Input: part model. Units: mm. Frame: model coordinates. Round coordinates to 2 decimals unless told otherwise and drop trailing zeros. Order: outer loops, then holes, each group sorted by start corner. A loop starts at its lowest first (then second) coordinate and runs counter-clockwise, first axis right, second up. Notation, with made-up numbers: (60.25, 75.25) -> (98.25, 75.25) arc R14 cw to (98.25, 79.25) -> close; hole circle Ø3 at (79, 7). An arc over 180 degrees is marked (long way). Use a Markdown table: item, result.
from build123d import *

# Parameters (mm, degrees)
F0_W     = 228.6
F0_H     = 177.8
F1_DEPTH = 3.175
F2_R     = 5.08


with BuildPart() as f1:
    # F0 (on Top) → F1 (new body)
    with BuildSketch(Plane.XY):
        with Locations((-0.871601, -3.897959)):
            Rectangle(F0_W, F0_H)
        Polygon((-35.42317, -63.4338), (-80.133474, -63.4338), (-56.54095, -14.745583), align=None, mode=Mode.SUBTRACT)
        Polygon((23.823941, -63.4338), (-13.718781, -63.4338), (4.465975, -14.745583), align=None, mode=Mode.SUBTRACT)
        Polygon((80.13803, -63.4338), (42.118688, -63.4338), (57.847038, -15.083696), align=None, mode=Mode.SUBTRACT)
        with BuildLine():
            Line((-90.692364, -63.4338), (-90.692364, 57.993443))
            Line((-90.692364, 57.993443), (-67.099841, 19.27751))
            ThreePointArc((-67.099841, 19.27751), (-62.324984, 2.265963), (-67.099841, -14.745583))
            Line((-67.099841, -14.745583), (-90.692364, -63.4338))
        make_face(mode=Mode.SUBTRACT)
        with BuildLine():
            ThreePointArc((-46.568668, -14.745583), (-50.040228, 2.291953), (-46.322669, 19.27751))
            Line((-46.322669, 19.27751), (-24.523671, 57.993443))
            Line((-24.523671, 57.993443), (-7.852732, 19.27751))
            ThreePointArc((-7.852732, 19.27751), (-4.872698, 2.265963), (-7.852732, -14.745583))
            Line((-7.852732, -14.745583), (-25.450888, -63.4338))
            Line((-25.450888, -63.4338), (-46.568668, -14.745583))
        make_face(mode=Mode.SUBTRACT)
        Polygon((-56.54095, 19.27751), (-80.133474, 57.993443), (-34.060732, 57.993443), align=None, mode=Mode.SUBTRACT)
        with BuildLine():
            Line((49.04796, -14.745583), (33.209621, -63.4338))
            Line((33.209621, -63.4338), (13.851655, -14.745583))
            ThreePointArc((13.851655, -14.745583), (10.593866, 2.265963), (13.851655, 19.27751))
            Line((13.851655, 19.27751), (33.31961, 57.993443))
            Line((33.31961, 57.993443), (49.04796, 19.27751))
            ThreePointArc((49.04796, 19.27751), (51.745333, 2.265963), (49.04796, -14.745583))
        make_face(mode=Mode.SUBTRACT)
        Polygon((4.465975, 19.27751), (-14.891991, 57.993443), (23.823941, 57.993443), align=None, mode=Mode.SUBTRACT)
        with BuildLine():
            Line((66.646114, 19.27751), (88.937106, 57.993443))
            Line((88.937106, 57.993443), (88.937106, -63.4338))
            Line((88.937106, -63.4338), (69.157515, -14.745583))
            ThreePointArc((69.157515, -14.745583), (65.224515, 2.06834), (66.646114, 19.27751))
        make_face(mode=Mode.SUBTRACT)
        Polygon((57.847038, 19.27751), (42.118688, 57.993443), (80.13803, 57.993443), align=None, mode=Mode.SUBTRACT)
    extrude(amount=F1_DEPTH)

    # F2
    f2_edges = [f1.edges().sort_by_distance(p)[0] for p in [
        (-90.692364, -63.4338, 1.5875),
        (-90.692364, 57.993443, 1.5875),
    ]]
    fillet(f2_edges, radius=F2_R)


solid = f1.part
1) Cut plane B-B on x = 2. Return loops of the section in (y, z) (3 decimals).
Answer key:
| item | result |
|---|---|
| outline | (-92.798, 0) -> (-63.434, 0) -> (-63.434, 3.175) -> (-92.798, 3.175) -> close; (-21.348, 0) -> (24.209, 0) -> (24.209, 3.175) -> (-21.348, 3.175) -> close; (57.993, 0) -> (85.002, 0) -> (85.002, 3.175) -> (57.993, 3.175) -> close |
2) Cut plane C-C on y = 13. Return loops of the section in (x, z) (3 decimals).
Answer key:
| item | result |
|---|---|
| outline | (-115.172, 0) -> (-90.692, 0) -> (-90.692, 3.175) -> (-115.172, 3.175) -> close; (-64.137, 0) -> (-48.574, 0) -> (-48.574, 3.175) -> (-64.137, 3.175) -> close; (-6.037, 0) -> (11.863, 0) -> (11.863, 3.175) -> (-6.037, 3.175) -> close; (50.688, 0) -> (65.497, 0) -> (65.497, 3.175) -> (50.688, 3.175) -> close; (88.937, 0) -> (113.428, 0) -> (113.428, 3.175) -> (88.937, 3.175) -> close |
3) Draft query along X for faces 1 (the face through (-73.973, -28.929, 1.565)), 2 (the face through (79.186, -39.431, 1.565)). Return one class per face: released by +X, released by -X, zero draft, split by the parting line, or undercut.
Answer key:
| item | result |
|---|---|
| face 1 | undercut |
| face 2 | undercut |
4) Ray query, probe 1 along X at (y, z) = (-11, 0.7); probe 2 along X at (y, z) = (4.5, 0.5); probe 3 along Y at (x, z) = (-42.5, 2.75). Return the intervals inside material, ascending.
Answer key:
| item | result |
|---|---|
| probe 1 | x = -115.17 to -90.69, -65.14 to -47.99, -6.66 to 12.55, 50.12 to 67.79, 88.94 to 113.43 |
| probe 2 | x = -115.17 to -90.69, -62.4 to -49.97, -4.92 to 10.65, 51.7 to 65.1, 88.94 to 113.43 |
| probe 3 | y = -92.8 to -63.43, -47.12 to -24.13, 26.07 to 43.46, 57.99 to 85 |
5) Cut plane D-D on x = -22. Return loops of the section in (y, z) (3 decimals).
Answer key:
| item | result |
|---|---|
| outline | (-92.798, 0) -> (-53.886, 0) -> (-53.886, 3.175) -> (-92.798, 3.175) -> close; (52.133, 0) -> (85.002, 0) -> (85.002, 3.175) -> (52.133, 3.175) -> close |
6) Cut plane A-A on y = -36. State how many separate pieces and enclosed holes the cut face has, and give its area (3 significant figures).
Answer key:
| item | result |
|---|---|
| separate pieces | 8 |
| enclosed holes | 0 |
| area | 350 mm^2 |
